Could you check a few things on this model? Use its own coordinates, in mm. A direction names the side the tool comes from. Round coordinates to 2 decimals unless told otherwise and drop trailing zeros. Write each loop counter-clockwise with the first axis right and the second up, starting at its lowest first coordinate (ties: lowest second). Pieces come first, ordered by that corner, then holes. Notation, with made-up numbers: (84, -13) -> (115, -13) arc R17 ccw to (115, 2) -> close; hole circle Ø10 at (28, 19.25). An arc over 180 degrees is marked (long way). Answer as CSV lines item,"result". Start each with the question number.
Q1. Imagine slicing it at A-A on x = -10. Please give me the cut outline in (y, z).
Q2. If I drill on line 1 (Y direction, x = 11, z = -0.4); line 2 (Z direction, x = 3.5, y = 2); line 3 (Y direction, x = -10, z = -0.2), over which ranges is the centre line in solid material (lowest first)? Write a range as [from, to].
Q3. If we mould it in two halves opening along Y, with no side actions, what happens to faces 4 (the cylindrical face through (10.2, 1.4, 8.2)), 5 (the cylindrical face through (-10.8, -0.6, -0.2)), 6 (the flat face through (-3, -4.5, 4)), 7 (the cylindrical face through (19, 0.1, -0.2))? For each: pulls with the +Y half, pulls with the -Y half, needs draft (parallel to the pull), parting line crosses it, or undercut.
Q4. Will these pins go through, and if not, where does the flat tip stop? pin 1 Ø2.5 at (x, z) = (-0.5, 5.5) entering from +Y; pin 2 Ø2.5 at (x, y) = (11, 2) entering from +Z.
Q5. Imagine slicing it at B-B on x = 11. Please give me the cut outline in (y, z).
Q6. For faces 1 (the cylindrical face through (2.752, -4.254, 2.213)), 2 (the flat face through (2, 2, 0)), 3 (the cylindrical face through (13.5, 0.07, -0.25)), which set-ups out of +Z, -Z, +X, -X, +Y, -Y let a thin tool reach every point of the face, with its end or its side?
Q7. Imagine slicing it at D-D on x = 7. Please give me the cut outline in (y, z), and give its area (4 significant figures).
Q8. Imagine slicing it at C-C on y = 0. Give the number of separate pieces and of enclosed holes in the cut face, and give its area (3 significant figures).
from build123d import *

# Parameters (mm, degrees)
SKETCH_2_R      = 1.5
SKETCH_2_R_2    = 1
EXTRUDE_1_DEPTH = 0.5
SKETCH_1_R      = 1.5
SKETCH_1_R_2    = 1
EXTRUDE_2_DEPTH = 0.5
EXTRUDE_4_DEPTH = 0.5
FILLET_1_R      = 2.5


with BuildPart() as part:
    # Sketch 2 → Extrude 1 (new body)
    with BuildSketch(Plane.XY.offset(8)):
        with BuildLine():
            Line((15, 4), (-15, 4))
            Line((-15, 4), (-15, -4))
            Line((-15, -4), (15, -4))
            ThreePointArc((15, -4), (19, 0), (15, 4))
        make_face()
        with Locations((15, 0)):
            Circle(SKETCH_2_R, mode=Mode.SUBTRACT)
        with Locations((11, -2)):
            Circle(SKETCH_2_R_2, mode=Mode.SUBTRACT)
        with Locations((11, 2)):
            Circle(SKETCH_2_R_2, mode=Mode.SUBTRACT)
        with Locations((2, 0)):
            Circle(SKETCH_2_R_2, mode=Mode.SUBTRACT)
        with Locations((-4, 0)):
            Circle(SKETCH_2_R_2, mode=Mode.SUBTRACT)
        with Locations((-10, 0)):
            Circle(SKETCH_2_R_2, mode=Mode.SUBTRACT)
    extrude(amount=EXTRUDE_1_DEPTH)



with BuildPart() as body_2:
    # Sketch 1 → Extrude 2 (new body)
    with BuildSketch(Plane.XY):
        with BuildLine():
            Line((-15, 4), (15, 4))
            ThreePointArc((15, 4), (19, 0), (15, -4))
            Line((15, -4), (-15, -4))
            Line((-15, -4), (-15, 4))
        make_face()
        with Locations((15, 0)):
            Circle(SKETCH_1_R, mode=Mode.SUBTRACT)
        with Locations((-10, 0)):
            Circle(SKETCH_1_R_2, mode=Mode.SUBTRACT)
        with Locations((-4, 0)):
            Circle(SKETCH_1_R_2, mode=Mode.SUBTRACT)
        with Locations((2, 0)):
            Circle(SKETCH_1_R_2, mode=Mode.SUBTRACT)
        with Locations((11, 2)):
            Circle(SKETCH_1_R_2, mode=Mode.SUBTRACT)
        with Locations((11, -2)):
            Circle(SKETCH_1_R_2, mode=Mode.SUBTRACT)
    extrude(amount=-EXTRUDE_2_DEPTH)


with BuildPart() as part_1:
    add(part.part)

    add(body_2.part)  # Extrude 4 merges body 2
    # Sketch 4 → Extrude 4 (add)
    with BuildSketch(Plane(origin=(0, -4, 0), x_dir=(1, 0, 0), z_dir=(0, 1, 0))):
        Polygon((-15, 0.5), (2, 0.5), (15, 0.5), (15, -1.5), (2, -1.5), (2, -6.5), (15, -6.5), (15, -8.5), (2, -8.5), (-15, -8.5), align=None)
    extrude(amount=-EXTRUDE_4_DEPTH)

    # Fillet 1
    fillet_1_edges = [part_1.edges().sort_by_distance(p)[0] for p in [
        (2, -4.25, 1.5),
        (2, -4.25, 6.5),
    ]]
    fillet(fillet_1_edges, radius=FILLET_1_R - 0.0001)  # a hair under: the kernel refuses the full size


solid = part_1.part
Checks:
1,outline,"(-4.5, -0.5) -> (-1, -0.5) -> (-1, 0) -> (-4, 0) -> (-4, 8) -> (-1, 8) -> (-1, 8.5) -> (-4.5, 8.5) -> close; (1, -0.5) -> (4, -0.5) -> (4, 0) -> (1, 0) -> close; (1, 8) -> (4, 8) -> (4, 8.5) -> (1, 8.5) -> close"
2,line 1,"[-4.5, -3], [-1, 1], [3, 4]"
2,line 2,"[-0.5, 0], [8, 8.5]"
2,line 3,"[-4.5, -1], [1, 4]"
3,face 4,"undercut"
3,face 5,"undercut"
3,face 6,"pulls with the -Y half"
3,face 7,"parting line crosses it"
4,pin 1,"y = -4"
4,pin 2,"z = 8.5"
5,outline,"(-4.5, -0.5) -> (-3, -0.5) -> (-3, 0) -> (-4, 0) -> (-4, 1.5) -> (-4.5, 1.5) -> close; (-4.5, 6.5) -> (-4, 6.5) -> (-4, 8) -> (-3, 8) -> (-3, 8.5) -> (-4.5, 8.5) -> close; (-1, -0.5) -> (1, -0.5) -> (1, 0) -> (-1, 0) -> close; (-1, 8) -> (1, 8) -> (1, 8.5) -> (-1, 8.5) -> close; (3, -0.5) -> (4, -0.5) -> (4, 0) -> (3, 0) -> close; (3, 8) -> (4, 8) -> (4, 8.5) -> (3, 8.5) -> close"
6,face 1,"+X, +Y, -Y"
6,face 2,"+X, -X, +Y"
6,face 3,"+Z, -Z"
7,outline,"(-4.5, -0.5) -> (4, -0.5) -> (4, 0) -> (-4, 0) -> (-4, 1.5) -> (-4.5, 1.5) -> close; (-4.5, 6.5) -> (-4, 6.5) -> (-4, 8) -> (4, 8) -> (4, 8.5) -> (-4.5, 8.5) -> close"
7,area,"10.00 mm^2"
8,separate pieces,"10"
8,enclosed holes,"0"
8,area,"25.0 mm^2"
